```python
from build123d import *

# Parameters (mm, degrees)
SKETCH1_W           = 150
SKETCH1_H           = 150
BOSS_EXTRUDE1_DEPTH = 12
SKETCH8_W           = 200
SKETCH8_H           = 200
CUT_EXTRUDE7_DEPTH  = 15
BOSS_EXTRUDE2_DEPTH = 12
SKETCH6_W           = 42
SKETCH6_H           = 42
CUT_EXTRUDE5_DEPTH  = 5
SKETCH9_R           = 4
SKETCH9_R_2         = 2.5
CUT_EXTRUDE8_DEPTH  = 15
SKETCH10_R          = 12
SKETCH10_R_2        = 1.25
CUT_EXTRUDE9_DEPTH  = 10
SKETCH12_R          = 2.5
SKETCH12_R_2        = 5
SKETCH12_R_3        = 1.5
CUT_EXTRUDE10_DEPTH = 20
SKETCH16_R          = 26
CUT_EXTRUDE11_DEPTH = 3
SKETCH17_R          = 5
CUT_EXTRUDE12_DEPTH = 3


with BuildPart() as part:
    # Sketch1 → Boss-Extrude1 (new body)
    with BuildSketch(Plane(origin=(0, 0, 0), x_dir=(1, 0, 0), z_dir=(0, 1, 0))):
        Rectangle(SKETCH1_W, SKETCH1_H)
    extrude(amount=BOSS_EXTRUDE1_DEPTH)

    # Sketch8 → Cut-Extrude7 (cut)
    with BuildSketch(Plane(origin=(0, 12, 0), x_dir=(1, 0, 0), z_dir=(0, 1, 0))):
        Rectangle(SKETCH8_W, SKETCH8_H)
        with BuildLine():
            Line((-48.989794856, 50), (-20, 50))
            Line((-20, 50), (-20, 56))
            Line((-20, 56), (20, 56))
            Line((20, 56), (20, 50))
            Line((20, 50), (48.989794856, 50))
            ThreePointArc((48.989794856, 50), (70, 0), (48.989794856, -50))
            Line((48.989794856, -50), (20, -50))
            Line((20, -50), (20, -56))
            Line((20, -56), (-20, -56))
            Line((-20, -56), (-20, -50))
            Line((-20, -50), (-48.989794856, -50))
            ThreePointArc((-48.989794856, -50), (-70, 0), (-48.989794856, 50))
        make_face(mode=Mode.SUBTRACT)
    extrude(amount=-CUT_EXTRUDE7_DEPTH, mode=Mode.SUBTRACT)

    # Sketch11 → Boss-Extrude2 (add)
    with BuildSketch(Plane(origin=(0, 12, 0), x_dir=(1, 0, 0), z_dir=(0, 1, 0))):
        with BuildLine():
            Line((48.989794856, 50), (78.989794856, 50))
            ThreePointArc((78.989794856, 50), (100, 0), (78.989794856, -50))
            Line((78.989794856, -50), (48.989794856, -50))
            ThreePointArc((48.989794856, -50), (70, 0), (48.989794856, 50))
        make_face()
    extrude(amount=-BOSS_EXTRUDE2_DEPTH)

    # Sketch6 → Cut-Extrude5 (cut)
    with BuildSketch(Plane(origin=(0, 12, 0), x_dir=(1, 0, 0), z_dir=(0, 1, 0))):
        with Locations((58.172158289, -29)):
            Rectangle(SKETCH6_W, SKETCH6_H)
    extrude(amount=-CUT_EXTRUDE5_DEPTH, mode=Mode.SUBTRACT)

    # Sketch9 → Cut-Extrude8 (cut)
    with BuildSketch(Plane(origin=(0, 12, 0), x_dir=(1, 0, 0), z_dir=(0, 1, 0))):
        with Locations(Location((-35, 35, 0), (0, 0, 270))):
            Circle(SKETCH9_R)
        with Locations(Location((-35, -35, 0), (0, 0, 270))):
            Circle(SKETCH9_R)
        with Locations(Location((-19, 35, 0), (0, 0, 270))):
            Circle(SKETCH9_R_2)
        with Locations(Location((-51, 35, 0), (0, 0, 270))):
            Circle(SKETCH9_R_2)
        with Locations(Location((-19, -35, 0), (0, 0, 270))):
            Circle(SKETCH9_R_2)
        with Locations(Location((-51, -35, 0), (0, 0, 270))):
            Circle(SKETCH9_R_2)
    extrude(amount=-CUT_EXTRUDE8_DEPTH, mode=Mode.SUBTRACT)

    # Sketch10 → Cut-Extrude9 (cut)
    with BuildSketch(Plane(origin=(0, 7, 0), x_dir=(1, 0, 0), z_dir=(0, 1, 0))):
        with Locations(Location((58.172158289, -29, 0), (0, 0, 270))):
            Circle(SKETCH10_R)
        with Locations(Location((42.672158289, -13.5, 0), (0, 0, 270))):
            Circle(SKETCH10_R_2)
        with Locations(Location((73.672158289, -13.5, 0), (0, 0, 270))):
            Circle(SKETCH10_R_2)
        with Locations(Location((42.672158289, -44.5, 0), (0, 0, 270))):
            Circle(SKETCH10_R_2)
        with Locations(Location((73.672158289, -44.5, 0), (0, 0, 270))):
            Circle(SKETCH10_R_2)
    extrude(amount=-CUT_EXTRUDE9_DEPTH, mode=Mode.SUBTRACT)

    # Sketch12 → Cut-Extrude10 (cut)
    with BuildSketch(Plane(origin=(0, 12, 0), x_dir=(1, 0, 0), z_dir=(0, 1, 0))):
        with Locations(Location((0, 18.25, 0), (0, 0, 270))):
            Circle(SKETCH12_R)
        with Locations(Location((0, -18.25, 0), (0, 0, 270))):
            Circle(SKETCH12_R)
        with Locations(Location((0, 0, 0), (0, 0, 270))):
            Circle(SKETCH12_R_2)
        with Locations(Location((18.25, 0, 0), (0, 0, 270))):
            Circle(SKETCH12_R)
        with Locations(Location((-18.25, 0, 0), (0, 0, 270))):
            Circle(SKETCH12_R)
        with Locations(Location((76, 10, 0), (0, 0, 270))):
            Circle(SKETCH12_R_3)
        with Locations(Location((60, 10, 0), (0, 0, 270))):
            Circle(SKETCH12_R_3)
        with Locations(Location((44, 10, 0), (0, 0, 270))):
            Circle(SKETCH12_R_3)
    extrude(amount=-CUT_EXTRUDE10_DEPTH, mode=Mode.SUBTRACT)

    # Sketch16 → Cut-Extrude11 (cut)
    with BuildSketch(Plane.XZ):
        with Locations(Location((0, 0, 0), (0, 0, 270))):
            Circle(SKETCH16_R)
    extrude(amount=-CUT_EXTRUDE11_DEPTH, mode=Mode.SUBTRACT)

    # Sketch17 → Cut-Extrude12 (cut)
    with BuildSketch(Plane.XZ.offset(-3)):
        with Locations(Location((0, 18.25, 0), (0, 0, 270))):
            Circle(SKETCH17_R)
        with Locations(Location((0, -18.25, 0), (0, 0, 270))):
            Circle(SKETCH17_R)
    extrude(amount=-CUT_EXTRUDE12_DEPTH, mode=Mode.SUBTRACT)


solid = part.part
```
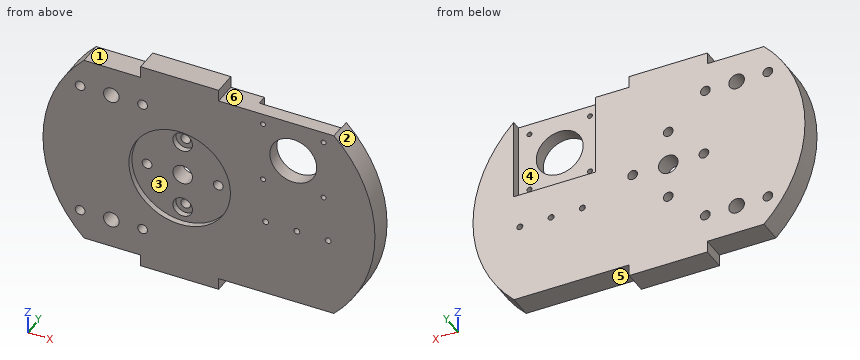
The model under review builds one solid part; all positions refer to its coordinate system, in mm. Face numbers are marked on the shaded views. A direction names the side the tool comes from. Round coordinates to 2 decimals unless told otherwise and drop trailing zeros. Loops run counter-clockwise (first coordinate to the right, second up) from the corner with the lowest first, then second, coordinate; pieces in that order, holes last. Notation, with made-up numbers: (51, 89.5) -> (67, 89.5) arc R20 ccw to (67, 121.5) -> close; hole circle Ø4 at (-5, 3). An arc over 180 degrees is marked (long way). Answer in a Markdown table with one row per item.
1) Tool access review of the marked faces 4, 5 and 6: name each direction out of +Z, -Z, +X, -X, +Y, -Y from which nothing blocks a thin tool from reaching the whole face with its end or side.
Taken from the geometry:
| item | result |
|---|---|
| face 4 | +Z, +Y |
| face 5 | -Z, +X, +Y, -Y |
| face 6 | +Z, +X, +Y, -Y |
2) Consider section A-A, the plane z = 35. Write out the cut boundary in (x, y).
Taken from the geometry:
| item | result |
|---|---|
| outline | (-60.62, 0) -> (-53.5, 0) -> (-53.5, 12) -> (-60.62, 12) -> close; (-48.5, 0) -> (-39, 0) -> (-39, 12) -> (-48.5, 12) -> close; (-31, 0) -> (-21.5, 0) -> (-21.5, 12) -> (-31, 12) -> close; (-16.5, 0) -> (47.78, 0) -> (47.78, 7) -> (37.17, 7) -> (37.17, 12) -> (-16.5, 12) -> close; (68.56, 0) -> (90.62, 0) -> (90.62, 12) -> (79.17, 12) -> (79.17, 7) -> (68.56, 7) -> close |
3) Consider section C-C, the plane y = 9.5. Count the separate pieces of the cut face and the enclosed holes in it, plus the area to 3 significant figures.
Taken from the geometry:
| item | result |
|---|---|
| separate pieces | 1 |
| enclosed holes | 14 |
| area | 14,100 mm² |
4) Consider section D-D, the plane x = 18.25. Write out the cut boundary in (y, z).
Taken from the geometry:
| item | result |
|---|---|
| outline | (0, -56) -> (12, -56) -> (12, -2.5) -> (3, -2.5) -> (3, -18.52) -> (0, -18.52) -> close; (0, 18.52) -> (3, 18.52) -> (3, 2.5) -> (12, 2.5) -> (12, 56) -> (0, 56) -> close |
5) Wall thickness on line 1 along X through (y, z) = (8.75, 0); line 2 along Z through (x, y) = (-34.5, 6.75); line 3 along X through (y, z) = (8.25, -37): over which ranges is each line inside the solid? List them lowest first.
Taken from the geometry:
| item | result |
|---|---|
| line 1 | x = -70 to -20.75, -15.75 to -5, 5 to 15.75, 20.75 to 100 |
| line 2 | z = -50 to -38.97, -31.03 to 31.03, 38.97 to 50 |
| line 3 | x = -59.42 to -52.5, -49.5 to -38.46, -31.54 to -20.5, -17.5 to 89.42 |
6) Draft analysis for pull direction X (two halves, no side actions). For the marked faces 1, 2 and 3, state which applies: pulls with the +X half, pulls with the -X half, needs draft (parallel to the pull), parting line crosses it, or undercut.
Taken from the geometry:
| item | result |
|---|---|
| face 1 | needs draft |
| face 2 | pulls with the +X half |
| face 3 | undercut |
7) Consider section B-B, the plane x = -24. Write out the cut boundary in (y, z), plus the area to 3 significant figures.
Taken from the geometry:
| item | result |
|---|---|
| outline | (0, -50) -> (12, -50) -> (12, 50) -> (0, 50) -> (0, 10) -> (3, 10) -> (3, -10) -> (0, -10) -> close |
| area | 1,140 mm² |
8) For pin 1 Ø6 at (x, z) = (0, 18.25) entering from -Y; pin 2 Ø1 at (x, y) = (75.5, 5) entering from -Z; pin 3 Ø6.5 at (y, z) = (4.5, 52.5) entering from +X, all flat-tipped, find the tip position at first contact; note any pin that passes through.
Taken from the geometry:
| item | result |
|---|---|
| pin 1 | stops at y = 6 |
| pin 2 | stops at z = -50 |
| pin 3 | stops at x = 79.74 |
